Work out the finished part from the listing and answer in its coordinate system (mm). A direction names the side the tool comes from. Give positions to 0.01 mm unless a question says otherwise; leave off trailing zeros. Write each loop counter-clockwise with the first axis right and the second up, starting at its lowest first coordinate (ties: lowest second). Pieces come first, ordered by that corner, then holes. Notation, with made-up numbers: (-24, -28) - (1, -28) arc R17 ccw to (1, -11) - close; hole circle Ø10 at (3, -5.5). An arc over 180 degrees is marked (long way). Write item = value, one per line.
from build123d import *

# Parameters (mm, degrees)
PAD_DEPTH       = 19.3
POCKET_DEPTH    = 12.301
POCKET002_DEPTH = 5
SKETCH003_R     = 1.5
POCKET003_DEPTH = 17.3
PAD001_DEPTH    = 12.3


with BuildPart() as part:
    # Sketch → Pad (new body)
    with BuildSketch(Plane.XY):
        Polygon((-9, 3.2), (-9, 9), (9, 9), (9, -9), (3.2, -9), align=None)
    extrude(amount=PAD_DEPTH)

    # Sketch001 (on DatumPlane) → Pocket (cut, through all)
    with BuildSketch(Plane.XY.offset(7)):
        Polygon((-9, 3.2), (3.2, 3.2), (3.2, -9), align=None)
    extrude(amount=POCKET_DEPTH, mode=Mode.SUBTRACT)

    # Sketch002 (on DatumPlane) → Pocket002 (cut)
    with BuildSketch(Plane.XY.offset(7)):
        with BuildLine():
            ThreePointArc((-2.168629, 0.268629), (-2.168629, 2.531371), (-4.431371, 2.531371))
            Line((-4.431371, 2.531371), (-6.694113, 0.268629))
            Line((-4.431371, -1.994113), (-6.694113, 0.268629))
            Line((-2.168629, 0.268629), (-4.431371, -1.994113))
        make_face()
        with BuildLine():
            ThreePointArc((2.531371, -4.431371), (2.531371, -2.168629), (0.268629, -2.168629))
            Line((0.268629, -2.168629), (-1.994113, -4.431371))
            Line((0.268629, -6.694113), (-1.994113, -4.431371))
            Line((2.531371, -4.431371), (0.268629, -6.694113))
        make_face()
    extrude(amount=-POCKET002_DEPTH, mode=Mode.SUBTRACT)

    # Sketch003 (on DatumPlane) → Pocket003 (cut)
    with BuildSketch(Plane.XY.offset(19.3)):
        with Locations((-3.3, 5)):
            Circle(SKETCH003_R)
        with Locations((5, -3.3)):
            Circle(SKETCH003_R)
    extrude(amount=-POCKET003_DEPTH, mode=Mode.SUBTRACT)

    # Sketch004 (on DatumPlane) → Pad001 (join)
    with BuildSketch(Plane.XY.offset(19.3)):
        with BuildLine():
            Line((-3.8, 3.2), (-2.8, 3.2))
            Line((-2.8, 3.2), (-2.8, 2.9))
            ThreePointArc((-2.8, 2.9), (-3.3, 2.985786), (-3.8, 2.9))
            Line((-3.8, 2.9), (-3.8, 3.2))
        make_face()
        with BuildLine():
            Line((3.2, -2.8), (2.9, -2.8))
            ThreePointArc((2.9, -3.8), (2.985786, -3.3), (2.9, -2.8))
            Line((2.9, -3.8), (3.2, -3.8))
            Line((3.2, -3.8), (3.2, -2.8))
        make_face()
    extrude(amount=-PAD001_DEPTH)


solid = part.part
1. Find section D-D, the plane z = 8.5. Give the vertices of the cut face in (x, y), then the cut area to 3 significant figures.
Solution:
outline = (-9, 3.2) - (-3.8, 3.2) - (-3.8, 2.9) arc R1.5 cw to (-2.8, 2.9) - (-2.8, 3.2) - (3.2, 3.2) - (3.2, -2.8) - (2.9, -2.8) arc R1.5 cw to (2.9, -3.8) - (3.2, -3.8) - (3.2, -9) - (9, -9) - (9, 9) - (-9, 9) - close; hole circle Ø3 at (-3.3, 5); hole circle Ø3 at (5, -3.3)
area = 162 mm^2
2. Straight lines are drawn through the part: line 1 (Y direction, x = -3.3, z = 5.5); line 2 (Y direction, x = 5, z = 10.5); line 3 (Y direction, x = -3.3, z = 8.25). For each, find the intervals that lie inside material, in ascending order.
Solution:
line_1 = -2.5 to -0.86, 3 to 3.5, 6.5 to 9
line_2 = -9 to -4.8, -1.8 to 9
line_3 = 2.99 to 3.5, 6.5 to 9
3. Given pin 1 (1.6 mm diameter, centred on x = -7.5, z = 15.5, fed in from -Y); pin 2 (1.6 mm diameter, centred on y = -7.5, z = 13, fed in from -X); pin 3 (3 mm diameter, centred on x = -6.5, y = 1.5, fed in from +Z), each flat-ended and moving along its own axis, determine where each tip first touches the part or whether it passes through.
Solution:
pin_1 = 3.2
pin_2 = 3.2
pin_3 = 7
4. For a pull along Y with two mould halves and no side action, classify faces 1 (the flat face through (2, 2, 0)), 2 (the flat face through (0, 9, 10)), 3 (the flat face through (-3, 5, 2)) as pulls with the +Y half, pulls with the -Y half, needs draft (parallel to the pull), parting line crosses it, or undercut.
Solution:
face_1 = needs draft
face_2 = pulls with the +Y half
face_3 = undercut
5. Find section B-B, the plane y = -0.75. Give the vertices of the cut face in (x, z).
Solution:
outline = (-5.05, 0) - (9, 0) - (9, 19.3) - (3.2, 19.3) - (3.2, 7) - (-3.19, 7) - (-3.19, 2) - (-5.05, 2) - close
6. Find section A-A, the plane z = 4.75. Give the vertices of the cut face in (x, y), then the cut area to 3 significant figures.
Solution:
outline = (-9, 3.2) - (-6.38, 0.58) - (-4.43, 2.53) arc R1.6 cw to (-2.17, 0.27) - (-4.12, -1.68) - (-1.68, -4.12) - (0.27, -2.17) arc R1.6 cw to (2.53, -4.43) - (0.58, -6.38) - (3.2, -9) - (9, -9) - (9, 9) - (-9, 9) - close; hole circle Ø3 at (-3.3, 5); hole circle Ø3 at (5, -3.3)
area = 210 mm^2
7. A tool of negligible diameter and unlimited length cuts with its end or side. For faces 4 (the cylindrical face through (2.986, -3.307, 13.236)), 5 (the cylindrical face through (-3.293, 2.986, 13.236)), 6 (the flat face through (2, -6, 7)), from which of +Z, -Z, +X, -X, +Y, -Y can it reach the whole face along a straight path? Write none if from no direction.
Solution:
face_4 = +Z, -X
face_5 = +Z, -Y
face_6 = +Z, -X, -Y
8. Find section C-C, the plane x = -5.75. Give the vertices of the cut face in (y, z), then the cut area to 3 significant figures.
Solution:
outline = (-0.05, 0) - (9, 0) - (9, 19.3) - (3.2, 19.3) - (3.2, 7) - (1.21, 7) - (1.21, 2) - (-0.05, 2) - close
area = 128 mm^2
